Read the model definition and answer for the solid it produces. Units are mm, in the model's axes. Give positions to 0.01 mm unless a question says otherwise; leave off trailing zeros. Order: outer loops, then holes, each group sorted by start corner. A loop starts at its lowest first (then second) coordinate and runs counter-clockwise, first axis right, second up. Notation, with made-up numbers: (-25, 74.5) - (17, 74.5) arc R16 cw to (17, 88.5) - close; hole circle Ø5 at (8.25, 37). An arc over 180 degrees is marked (long way). Write each question's results on one line, items separated by ' | '.
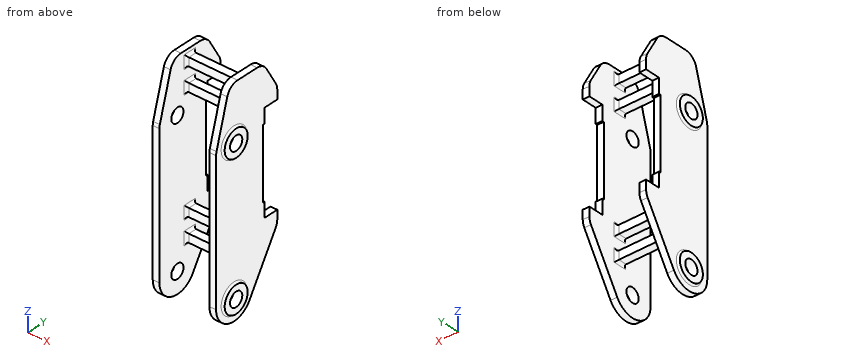
from build123d import *

# Parameters (mm, degrees)
SZKIC1_R                    = 8.5
DODANIE_WYCI_GNI_CIE1_DEPTH = 8
SZKIC2_R                    = 16
SZKIC2_R_2                  = 8.5
DODANIE_WYCI_GNI_CIE2_DEPTH = 2.5
ZAOKR_GLENIE1_R             = 2
DODANIE_WYCI_GNI_CIE3_REACH = 240.506
SZKIC3_W                    = 10
SZKIC3_H                    = 10
ZAOKR_GLENIE2_R             = 3


with BuildPart() as part:
    # Szkic1 → Dodanie-wyci_gni_cie1 (new body)
    with BuildSketch(Plane(origin=(0, 0, 0), x_dir=(0, 0, -1), z_dir=(1, 0, 0))):
        with BuildLine():
            Line((0, 0), (-10.980762114, 0))
            ThreePointArc((-10.980762114, 0), (-14.86304779, -0.511112606), (-18.480762114, -2.009618943))
            Line((-18.480762114, -2.009618943), (-41.1, -15.068842026))
            ThreePointArc((-41.1, -15.068842026), (-46.590381057, -20.559223083), (-48.6, -28.059223083))
            Line((-48.6, -28.059223083), (-48.6, -55.049432524))
            ThreePointArc((-48.6, -55.049432524), (-45.579532651, -64.076657871), (-37.734560337, -69.468357963))
            Line((-37.734560337, -69.468357963), (14.404264621, -84.418925439))
            ThreePointArc((14.404264621, -84.418925439), (16.451228444, -84.854021031), (18.538824959, -85))
            Line((18.538824959, -85), (186.430712438, -85))
            ThreePointArc((186.430712438, -85), (210.491878328, -66.703464298), (199.290846236, -38.627855618))
            Line((199.290846236, -38.627855618), (138.569001646, -2.142490489))
            ThreePointArc((138.569001646, -2.142490489), (134.852006163, -0.545543202), (130.843430522, 0))
            Line((130.843430522, 0), (120.003298683, 0))
            Line((120.003298683, 0), (120.003298683, -18))
            Line((120.003298683, -18), (102.303298683, -18))
            Line((102.303298683, -18), (102.303298683, -20))
            Line((102.303298683, -20), (17.7, -20))
            Line((17.7, -20), (17.7, -18))
            Line((17.7, -18), (0, -18))
            Line((0, -18), (0, 0))
        make_face()
        with Locations((16.430712438, -60)):
            Circle(SZKIC1_R, mode=Mode.SUBTRACT)
        with Locations((186.430712438, -60)):
            Circle(SZKIC1_R, mode=Mode.SUBTRACT)
    extrude(amount=DODANIE_WYCI_GNI_CIE1_DEPTH)

    # Szkic2 → Dodanie-wyci_gni_cie2 (add)
    # profile 1 of 2: a face of its own
    with BuildSketch(Plane(origin=(8, 0, 0), x_dir=(0, 0, -1), z_dir=(1, 0, 0))):
        with Locations((16.430712438, -60)):
            Circle(SZKIC2_R)
        with Locations((16.430712438, -60)):
            Circle(SZKIC2_R_2, mode=Mode.SUBTRACT)
    # profile 2 of 2: a face of its own
    with BuildSketch(Plane(origin=(8, 0, 0), x_dir=(0, 0, -1), z_dir=(1, 0, 0))):
        with Locations((186.430712438, -60)):
            Circle(SZKIC2_R)
        with Locations((186.430712438, -60)):
            Circle(SZKIC2_R_2, mode=Mode.SUBTRACT)
    extrude(amount=DODANIE_WYCI_GNI_CIE2_DEPTH)

    # Zaokr_glenie1
    zaokr_glenie1_edges = [part.edges().sort_by_distance(p)[0] for p in [
        (8, -60, -0.430712438),
        (8, -60, -170.430712438),
    ]]
    fillet(zaokr_glenie1_edges, radius=ZAOKR_GLENIE1_R)


with BuildPart() as body_2:
    # Lustro3: mirrored copy
    add(part.part.mirror(Plane.ZY.offset(30)))

    # Szkic3 → Dodanie-wyci_gni_cie3 (add, up to next)
    with BuildSketch(Plane.ZY, mode=Mode.PRIVATE) as dodanie_wyci_gni_cie3_sk1:
        with Locations((8.6, -42.5)):
            Rectangle(SZKIC3_W, SZKIC3_H)
    dodanie_wyci_gni_cie3_tool1 = extrude(dodanie_wyci_gni_cie3_sk1.sketch, amount=DODANIE_WYCI_GNI_CIE3_REACH, mode=Mode.PRIVATE) - body_2.part
    # Szkic3 → Dodanie-wyci_gni_cie3 (add, up to next)
    with BuildSketch(Plane.ZY, mode=Mode.PRIVATE) as dodanie_wyci_gni_cie3_sk2:
        with Locations((36.6, -42.5)):
            Rectangle(SZKIC3_W, SZKIC3_H)
    dodanie_wyci_gni_cie3_tool2 = extrude(dodanie_wyci_gni_cie3_sk2.sketch, amount=DODANIE_WYCI_GNI_CIE3_REACH, mode=Mode.PRIVATE) - body_2.part
    # Szkic3 → Dodanie-wyci_gni_cie3 (add, up to next)
    with BuildSketch(Plane.ZY, mode=Mode.PRIVATE) as dodanie_wyci_gni_cie3_sk3:
        with Locations((-155.4, -42.5)):
            Rectangle(SZKIC3_W, SZKIC3_H)
    dodanie_wyci_gni_cie3_tool3 = extrude(dodanie_wyci_gni_cie3_sk3.sketch, amount=DODANIE_WYCI_GNI_CIE3_REACH, mode=Mode.PRIVATE) - body_2.part
    # Szkic3 → Dodanie-wyci_gni_cie3 (add, up to next)
    with BuildSketch(Plane.ZY, mode=Mode.PRIVATE) as dodanie_wyci_gni_cie3_sk4:
        with Locations((-127.4, -42.5)):
            Rectangle(SZKIC3_W, SZKIC3_H)
    dodanie_wyci_gni_cie3_tool4 = extrude(dodanie_wyci_gni_cie3_sk4.sketch, amount=DODANIE_WYCI_GNI_CIE3_REACH, mode=Mode.PRIVATE) - body_2.part

    add(part.part)  # Dodanie-wyci_gni_cie3 merges part
    add(dodanie_wyci_gni_cie3_tool1.solids().sort_by_distance((0, -42.5, 8.6))[0])
    add(dodanie_wyci_gni_cie3_tool2.solids().sort_by_distance((0, -42.5, 36.6))[0])
    add(dodanie_wyci_gni_cie3_tool3.solids().sort_by_distance((0, -42.5, -155.4))[0])
    add(dodanie_wyci_gni_cie3_tool4.solids().sort_by_distance((0, -42.5, -127.4))[0])

    # Zaokr_glenie2
    zaokr_glenie2_edges = [body_2.edges().sort_by_distance(p)[0] for p in [
        (-60, -42.5, 31.6),
        (-60, -47.5, 36.6),
        (-60, -42.5, 41.6),
        (-60, -37.5, 36.6),
        (0, -47.5, 36.6),
        (0, -42.5, 31.6),
        (0, -42.5, 41.6),
        (0, -37.5, 36.6),
        (-60, -42.5, -160.4),
        (-60, -47.5, -155.4),
        (-60, -42.5, -150.4),
        (-60, -37.5, -155.4),
        (0, -42.5, -160.4),
        (0, -47.5, -155.4),
        (0, -42.5, -150.4),
        (0, -37.5, -155.4),
        (-60, -42.5, -132.4),
        (-60, -47.5, -127.4),
        (-60, -42.5, -122.4),
        (-60, -37.5, -127.4),
        (0, -47.5, -127.4),
        (0, -42.5, -132.4),
        (0, -42.5, -122.4),
        (0, -37.5, -127.4),
        (-60, -42.5, 3.6),
        (-60, -47.5, 8.6),
        (-60, -42.5, 13.6),
        (-60, -37.5, 8.6),
        (0, -47.5, 8.6),
        (0, -42.5, 3.6),
        (0, -42.5, 13.6),
        (0, -37.5, 8.6),
    ]]
    fillet(zaokr_glenie2_edges, radius=ZAOKR_GLENIE2_R)


solid = body_2.part
(1) Section B-B (x = -27) is taken. Give the vertices of the cut face in (y, z), plus the area to 3 significant figures.
Conclusion:
outline: (-47.5, -160.4) - (-37.5, -160.4) - (-37.5, -150.4) - (-47.5, -150.4) - close; (-47.5, -132.4) - (-37.5, -132.4) - (-37.5, -122.4) - (-47.5, -122.4) - close; (-47.5, 3.6) - (-37.5, 3.6) - (-37.5, 13.6) - (-47.5, 13.6) - close; (-47.5, 31.6) - (-37.5, 31.6) - (-37.5, 41.6) - (-47.5, 41.6) - close | area: 400 mm^2
(2) Each of these flat-tipped pins is pushed along its axis until it touches: pin 1 (11 mm diameter, centred on x = -32, y = -44.5, fed in from -Z); pin 2 (6.5 mm diameter, centred on x = 2.5, y = -5.5, fed in from -Z); pin 3 (9 mm diameter, centred on x = -65.5, z = -113.5, fed in from +Y). Where does it stop, or does it pass through?
Conclusion:
pin 1: z = -160.4 | pin 2: z = -149.57 | pin 3: y = -18
(3) Section D-D (x = -63.5) is taken. Give the vertices of the cut face in (y, z).
Conclusion:
outline: (-85, -186.43) arc R24.97 ccw to (-38.63, -199.29) - (-2.14, -138.57) arc R15 ccw to (0, -130.84) - (0, -120) - (-18, -120) - (-18, -102.3) - (-20, -102.3) - (-20, -17.7) - (-18, -17.7) - (-18, 0) - (0, 0) - (0, 10.98) arc R15 ccw to (-2.01, 18.48) - (-15.07, 41.1) arc R15 ccw to (-28.06, 48.6) - (-55.05, 48.6) arc R15 ccw to (-69.47, 37.73) - (-84.42, -14.4) arc R15 ccw to (-85, -18.54) - close; hole circle Ø17 at (-60, -186.43); hole circle Ø17 at (-60, -16.43)
(4) Section C-C (y = -32) is taken. Give the vertices of the cut face in (x, z).
Conclusion:
outline: (-68, -188.26) - (-60, -188.26) - (-60, 48.6) - (-68, 48.6) - close; (0, -188.26) - (8, -188.26) - (8, 48.6) - (0, 48.6) - close
(5) Section A-A (z = -62) is taken. Give the vertices of the cut face in (x, y), plus the area to 3 significant figures.
Conclusion:
outline: (-68, -85) - (-60, -85) - (-60, -20) - (-68, -20) - close; (0, -85) - (8, -85) - (8, -20) - (0, -20) - close | area: 1,040 mm^2
(6) Consider probe 1 along X at (y, z) = (-56, -194); probe 2 along X at (y, z) = (-31, -104); probe 3 along Y at (x, z) = (-66.5, -165). Determine where each line is inside the solid, lowest interval first. Write a range as [from, to].
Conclusion:
probe 1: [-70.5, -60], [0, 10.5] | probe 2: [-68, -60], [0, 8] | probe 3: [-85, -18.02]
